Source: three-view drawing plus pictorial views. Frame: mm from the lowest corner of the part. A direction names the side the tool comes from. Give positions to 0.01 mm unless a question says otherwise; leave off trailing zeros. Order: outer loops, then holes, each group sorted by start corner. A loop starts at its lowest first (then second) coordinate and runs counter-clockwise, first axis right, second up. Notation, with made-up numbers: M -5.5,58.25 L 8.5,58.25 A31 cw 8.5,83.25 Z; hole C -18,-40 d11. An arc over 180 degrees is marked long. Use CSV: the item, a comma, the result in double quotes. Start each with the question number.
1. Reachability of the marked faces 1 and 2 from +Z, -Z, +X, -X, +Y, -Y: full face, straight path, thin tool, end or side. Return the list, or none.
2. Section query A-A, the plane z = 7.5. Return the cut outline in (x, y).
3. Pin query (flat end, axial travel): P1, Ø1, axis at y = 9.5, z = 11, coming from the -X side; P2, Ø6, axis at x = 7.5, y = 12.5, coming from the -Z side; P3, Ø5, axis at y = 6, z = 4.5, coming from the +X side; P4, Ø4, axis at x = 6, z = 6, coming from the -Y side. Return the tip coordinate at first contact, or that it passes through.
4. Section query C-C, the plane z = 2.5. Return the cut outline in (x, y), plus the area to 3 significant figures.
5. Section query B-B, the plane y = 20. Return the cut outline in (x, z), plus the area to 3 significant figures.
6. Mould query, pull axis Z, two halves, no side actions, for the marked faces 3, 4, 5 and 6. Classes: released by +Z, released by -Z, zero draft, split by the parting line, or undercut.
7. Line query: line 1 along Z through (x, y) = (6, 14.5); line 2 along Y through (x, z) = (11.75, 10); line 3 along Z through (x, y) = (5.5, 26.25) (1 decimal). Output: solid intervals per line, ascending. Write a range as [from, to].
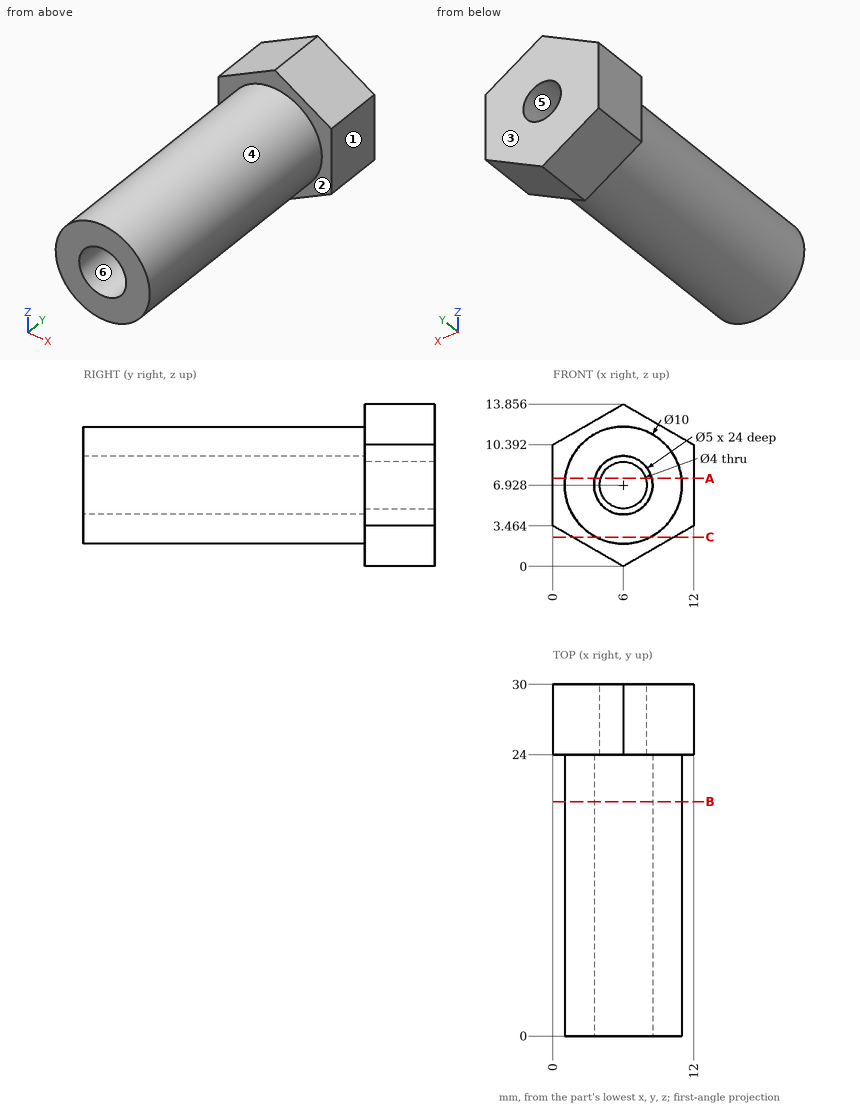
Result set:
1,face 1,"+Z, -Z, +X, +Y, -Y"
1,face 2,"-Y"
2,outline,"M 0,24 L 1.03,24 L 1.03,0 L 3.57,0 L 3.57,24 L 4.08,24 L 4.08,30 L 0,30 Z; M 7.92,24 L 8.43,24 L 8.43,0 L 10.97,0 L 10.97,24 L 12,24 L 12,30 L 7.92,30 Z"
3,P1,"x = 2.5"
3,P2,"z = 1.93"
3,P3,"x = 11"
3,P4,"y = 0"
4,outline,"M 1.67,24 L 3.68,24 L 3.68,0 L 8.32,0 L 8.32,24 L 10.33,24 L 10.33,30 L 1.67,30 Z"
4,area,"163 mm2"
5,outline,"C 6,6.93 d10; hole C 6,6.93 d5"
5,area,"58.9 mm2"
6,face 3,"zero draft"
6,face 4,"split by the parting line"
6,face 5,"undercut"
6,face 6,"undercut"
7,line 1,"[1.93, 4.43], [9.43, 11.93]"
7,line 2,"[24, 30]"
7,line 3,"[0.3, 5], [8.9, 13.6]"
